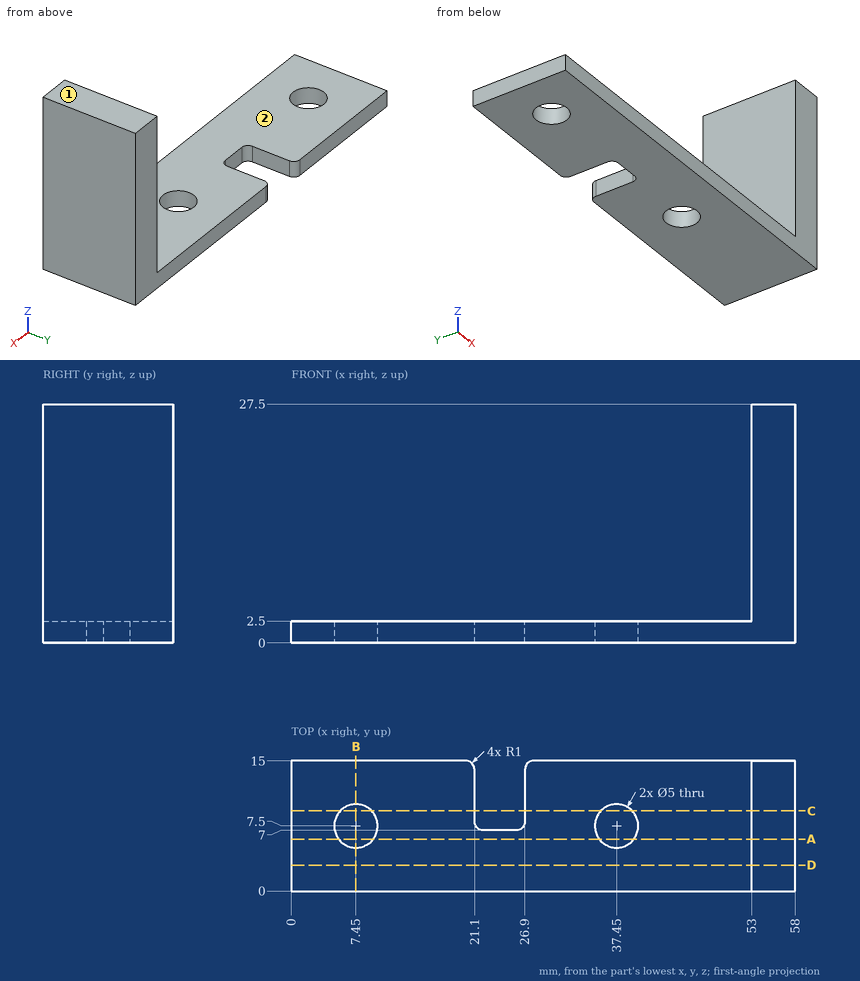
Geometry: see drawing. Coordinates: mm, zero at the bounding-box minimum. A direction names the side the tool comes from. Give positions to 0.01 mm unless a question says otherwise; leave off trailing zeros. Loops run counter-clockwise (first coordinate to the right, second up) from the corner with the lowest first, then second, coordinate; pieces in that order, holes last. Notation, with made-up numbers: M 71,87.5 L 103,87.5 A28 ccw 103,124.5 Z; hole C 9,1.25 d10. An arc over 180 degrees is marked long. Use one line per item in the form item = value.
1. Section query C-C, the plane y = 9.25. Return the cut outline in (x, z).
Numbers:
outline = M 0,0 L 5.66,0 L 5.66,2.5 L 0,2.5 Z; M 9.24,0 L 21.1,0 L 21.1,2.5 L 9.24,2.5 Z; M 26.9,0 L 35.66,0 L 35.66,2.5 L 26.9,2.5 Z; M 39.24,0 L 58,0 L 58,27.5 L 53,27.5 L 53,2.5 L 39.24,2.5 Z
2. Reachability of the marked faces 1 and 2 from +Z, -Z, +X, -X, +Y, -Y: full face, straight path, thin tool, end or side. Return the list, or none.
Numbers:
face_1 = +Z, +X, -X, +Y, -Y
face_2 = +Z, -X, +Y, -Y
3. First-contact query: pin 1 (3 mm diameter, centred on x = 24.5, z = 1, fed in from +Y) (3 decimals); pin 2 (4 mm diameter, centred on x = 7.45, y = 7.5, fed in from -Z); pin 3 (7.5 mm diameter, centred on x = 37.5, y = 6, fed in from +Z). Flat tips, straight axial feed; report the tip coordinate or a pass-through.
Numbers:
pin_1 = 7.005
pin_2 = through
pin_3 = 2.5
4. Section query A-A, the plane y = 6. Return the cut outline in (x, z), and give its area (3 significant figures).
Numbers:
outline = M 0,0 L 5.45,0 L 5.45,2.5 L 0,2.5 Z; M 9.45,0 L 35.45,0 L 35.45,2.5 L 9.45,2.5 Z; M 39.45,0 L 58,0 L 58,27.5 L 53,27.5 L 53,2.5 L 39.45,2.5 Z
area = 250 mm²
5. Line query: L1, parallel to Y at x = 7.45, z = 0.8; L2, parallel to X at y = 7.25, z = 1.25; L3, parallel to Z at x = 46.5, y = 3.5. Output: solid intervals per line, ascending.
Numbers:
L1 = 0 to 5, 10 to 15
L2 = 0 to 4.96, 9.94 to 21.44, 26.56 to 34.96, 39.94 to 58
L3 = 0 to 2.5
6. Section query D-D, the plane y = 3. Return the cut outline in (x, z), and give its area (3 significant figures).
Numbers:
outline = M 0,0 L 58,0 L 58,27.5 L 53,27.5 L 53,2.5 L 0,2.5 Z
area = 270 mm²
7. Section query B-B, the plane x = 7.45. Return the cut outline in (y, z).
Numbers:
outline = M 0,0 L 5,0 L 5,2.5 L 0,2.5 Z; M 10,0 L 15,0 L 15,2.5 L 10,2.5 Z
